```python
from build123d import *

# Parameters (mm, degrees)
F1_DEPTH = 25.4
F2_W     = 72.5054554641
F2_H     = 12.4690914527
F3_DEPTH = 25.4
F5_DEPTH = 72.39
F6_R     = 3.324206073
F7_DEPTH = 107.4789683862
F9_DEPTH = 21.4076038046


with BuildPart() as f1:
    # F0 (on Top) → F1 (new body)
    with BuildSketch(Plane.XY):
        with BuildLine():
            Line((55.0140924752, 15.1534089819), (-52.9936365783, 15.1534089819))
            ThreePointArc((-52.9936365783, 15.1534089819), (-70.3016052161, 0), (-52.9936365783, -15.1534089819))
            Line((-52.9936365783, -15.1534089819), (55.0140924752, -15.1534089819))
            ThreePointArc((55.0140924752, -15.1534089819), (70.167501457, 0), (55.0140924752, 15.1534089819))
        make_face()
        with BuildLine():
            ThreePointArc((-55.0140924752, -7.3239727508), (-62.338065226, 0), (-55.0140924752, 7.3239727508))
            ThreePointArc((-55.0140924752, 7.3239727508), (-49.8352616778, 5.1788307973), (-47.6901197244, 0))
            ThreePointArc((-47.6901197244, 0), (-49.8352616778, -5.1788307973), (-55.0140924752, -7.3239727508))
        make_face(mode=Mode.SUBTRACT)
        with BuildLine():
            ThreePointArc((55.0140924752, -7.1054389054), (47.9086535698, 0), (55.0140924752, 7.1054389054))
            ThreePointArc((55.0140924752, 7.1054389054), (60.0383965085, 5.0243040333), (62.1195313806, 0))
            ThreePointArc((62.1195313806, 0), (60.0383965085, -5.0243040333), (55.0140924752, -7.1054389054))
        make_face(mode=Mode.SUBTRACT)
    extrude(amount=F1_DEPTH)

    # F2 (on face) → F3 (join)
    with BuildSketch(Plane.XY.offset(25.4)):
        with Locations((0.9236354381, -0.1154546626)):
            Rectangle(F2_W, F2_H)
    extrude(amount=F3_DEPTH)

    # F4 (on face) → F5 (join)
    with BuildSketch(Plane.YZ.offset(37.1763631701)):
        with BuildLine():
            Line((3.0379533135, 50.8), (5.9346302823, 50.8))
            ThreePointArc((5.9346302823, 50.8), (-0.1154546626, 56.8500849449), (-6.1655396075, 50.8))
            Line((-6.1655396075, 50.8), (-3.2688626387, 50.8))
            ThreePointArc((-3.2688626387, 50.8), (-0.1154546626, 53.9534079761), (3.0379533135, 50.8))
        make_face()
    extrude(amount=-F5_DEPTH)

    # F6 (on face) → F7 (cut, through all)
    with BuildSketch(Plane.YZ.offset(37.1763631701)):
        with Locations((0, 50.8)):
            Circle(F6_R)
        with BuildLine():
            ThreePointArc((-3.2688626387, 50.8), (-0.1154546626, 53.9534079761), (3.0379533135, 50.8))
            Line((3.0379533135, 50.8), (-3.2688626387, 50.8))
        make_face(mode=Mode.SUBTRACT)
    extrude(amount=-F7_DEPTH, mode=Mode.SUBTRACT)

    # F8 (on face) → F9 (cut, through all)
    with BuildSketch(Plane(origin=(0, 6.1190910637, 0), x_dir=(-1, 0, 0), z_dir=(0, 1, 0))):
        with BuildLine():
            Line((25.97059982, 50.8), (-25.97059982, 50.8))
            ThreePointArc((-25.97059982, 50.8), (0, 30.2373519431), (25.97059982, 50.8))
        make_face()
        with BuildLine():
            ThreePointArc((25.97059982, 50.8), (26.5033603392, 53.8389546874), (26.681742232, 56.9190941751))
            ThreePointArc((26.681742232, 56.9190941751), (-3.0801394877, 83.4224545143), (-25.97059982, 50.8))
            Line((-25.97059982, 50.8), (25.97059982, 50.8))
        make_face()
    extrude(amount=-F9_DEPTH, mode=Mode.SUBTRACT)


solid = f1.part
```
Verification items for the finished model (mm, model axes). A direction names the side the tool comes from. Coordinates: 2 decimals unless noted, no trailing zeros. Loops run counter-clockwise (first coordinate to the right, second up) from the corner with the lowest first, then second, coordinate; pieces in that order, holes last. Notation, with made-up numbers: (71, -26.5) - (82, -26.5) arc R24 cw to (82, 1.5) - close; hole circle Ø6 at (-2, 75). An arc over 180 degrees is marked (long way). Return JSON: item names as keys, results as strings.
1. Section check C-C, the plane z = 41. Record the boundary of the cut face in (x, y).
Established:
{"outline": "(-35.33, -6.35) - (-21.41, -6.35) - (-21.41, 6.12) - (-35.33, 6.12) - close; (21.41, -6.35) - (37.18, -6.35) - (37.18, 6.12) - (21.41, 6.12) - close"}
2. Go/stop test with flat-tipped pins: pin 1 (13.5 mm diameter, centred on y = -2.5, z = 35, fed in from -X); pin 2 (7.5 mm diameter, centred on x = -25.5, z = 16.5, fed in from -Y); pin 3 (1.5 mm diameter, centred on x = -32.5, y = -5.5, fed in from +Z); pin 4 (4 mm diameter, centred on y = -1.5, z = 14.5, fed in from +X). Record where each tip stops, or that it passes through.
Established:
{"pin 1": "stops at x = -35.33", "pin 2": "stops at y = -15.15", "pin 3": "stops at z = 54.69", "pin 4": "stops at x = 70.17"}
3. Mould release check, pull along Y, two halves, no side actions. Record for faces 1 (the cylindrical face through (-30.069, -0.721, 47.555)), 2 (the cylindrical face through (-30.53, 0.02, 56.85)), 3 (the flat face through (0, -6.35, 29)): +Y half, -Y half, draft (parallel to the pull), parting line (faces both ways), or undercut.
Established:
{"face 1": "undercut", "face 2": "parting line", "face 3": "-Y half"}
4. Tool access check on faces 4 (the flat face through (0, 6.119, 29)), 5 (the flat face through (0, -15.153, 13)), 6 (the flat face through (37.176, 0, 41)), 7 (the flat face through (-35.214, 0, 55)). Record the directions out of +Z, -Z, +X, -X, +Y, -Y that give a thin tool (end or side, any length) a straight path to the whole face; none if there is none.
Established:
{"face 4": "+Z, +X, -X, +Y", "face 5": "+Z, -Z, +X, -Y", "face 6": "+Z, +X, +Y, -Y", "face 7": "+Z, -X, +Y, -Y"}
5. Thickness scan on L1, parallel to Z at x = -27.75, y = 0; L2, parallel to X at y = -5, z = 16.5; L3, parallel to X at y = 1, z = 21.5. Record the ranges inside material, lowest first.
Established:
{"L1": "z = 0 to 47.48, 54.12 to 56.85", "L2": "x = -69.46 to -60.37, -49.66 to 49.97, 60.06 to 69.32", "L3": "x = -70.27 to -62.27, -47.76 to 47.98, 62.05 to 70.13"}
6. Section check D-D, the plane x = -37.5. Record the boundary of the cut face in (y, z), then the cut area to 3 significant figures.
Established:
{"outline": "(-15.15, 0) - (15.15, 0) - (15.15, 25.4) - (-15.15, 25.4) - close", "area": "770 mm2"}
7. Section check A-A, the plane z = 13. Record the boundary of the cut face in (x, y).
Established:
{"outline": "(-52.99, -15.15) - (55.01, -15.15) arc R15.15 ccw to (55.01, 15.15) - (-52.99, 15.15) arc R15.29 ccw (long way) to start; hole circle Ø14.65 at (-55.01, 0); hole circle Ø14.21 at (55.01, 0)"}
8. Section check B-B, the plane x = 59. Record the boundary of the cut face in (y, z).
Established:
{"outline": "(-14.62, 0) - (-5.88, 0) - (-5.88, 25.4) - (-14.62, 25.4) - close; (5.88, 0) - (14.62, 0) - (14.62, 25.4) - (5.88, 25.4) - close"}
